Could you check a few things on this model? Use its own coordinates, in mm. A direction names the side the tool comes from. Coordinates: 2 decimals unless noted, no trailing zeros. Loops run counter-clockwise (first coordinate to the right, second up) from the corner with the lowest first, then second, coordinate; pieces in that order, holes last.
from build123d import *

# Parameters (mm, degrees)
SKETCH1_R           = 34
SKETCH1_R_2         = 31.5
BOSS_EXTRUDE1_DEPTH = 13
SKETCH2_R           = 34
BOSS_EXTRUDE2_DEPTH = 3
FILLET1_R           = 3
SKETCH3_R           = 2.5
SKETCH3_R_2         = 1.5
BOSS_EXTRUDE3_DEPTH = 10
SKETCH5_R           = 32.5
SKETCH5_R_2         = 31.5
CUT_EXTRUDE1_DEPTH  = 3
SKETCH6_R           = 1.6
CUT_EXTRUDE2_DEPTH  = 0.4
SKETCH7_R           = 1.5
CUT_EXTRUDE3_DEPTH  = 16.6


with BuildPart() as part:
    # Sketch1 → Boss-Extrude1 (new body)
    with BuildSketch(Plane.XY):
        Circle(SKETCH1_R)
        Circle(SKETCH1_R_2, mode=Mode.SUBTRACT)
    extrude(amount=BOSS_EXTRUDE1_DEPTH)

    # Sketch2 → Boss-Extrude2 (add)
    with BuildSketch(Plane.XY.offset(13)):
        Circle(SKETCH2_R)
    extrude(amount=BOSS_EXTRUDE2_DEPTH)

    # Fillet1
    fillet1_edges = [part.edges().sort_by_distance(p)[0] for p in [
        (-34, 0, 16),
    ]]
    fillet(fillet1_edges, radius=FILLET1_R)

    # Sketch3 → Boss-Extrude3 (add)
    with BuildSketch(Plane(origin=(0, 0, 13), x_dir=(-1, 0, 0), z_dir=(0, 0, -1))):
        with Locations((-20, 0)):
            Circle(SKETCH3_R)
        with Locations((-20, 0)):
            Circle(SKETCH3_R_2, mode=Mode.SUBTRACT)
        with Locations((20, 0)):
            Circle(SKETCH3_R)
        with Locations((20, 0)):
            Circle(SKETCH3_R_2, mode=Mode.SUBTRACT)
    extrude(amount=BOSS_EXTRUDE3_DEPTH)

    # Sketch5 → Cut-Extrude1 (cut)
    with BuildSketch(Plane(origin=(0, 0, 0), x_dir=(-1, 0, 0), z_dir=(0, 0, -1))):
        Circle(SKETCH5_R)
        Circle(SKETCH5_R_2, mode=Mode.SUBTRACT)
    extrude(amount=-CUT_EXTRUDE1_DEPTH, mode=Mode.SUBTRACT)

    # Sketch6 → Cut-Extrude2 (cut)
    with BuildSketch(Plane.XY.offset(16)):
        with Locations((0, -25)):
            Circle(SKETCH6_R)
    extrude(amount=-CUT_EXTRUDE2_DEPTH, mode=Mode.SUBTRACT)

    # Sketch7 → Cut-Extrude3 (cut, through all)
    with BuildSketch(Plane.XY.offset(15.6)):
        with Locations((0, -25)):
            Circle(SKETCH7_R)
    extrude(amount=-CUT_EXTRUDE3_DEPTH, mode=Mode.SUBTRACT)


solid = part.part
(1) For pin 1 (4 mm diameter, centred on x = -20, y = 0, fed in from -Z); pin 2 (19.5 mm diameter, centred on x = 3, y = 11, fed in from -Z); pin 3 (1.5 mm diameter, centred on x = 9.5, z = 3, fed in from -Y), each with a flat end and sliding along its axis, tell me the tip position at first contact or that it passes through.
Answers:
pin 1: stops at z = 3
pin 2: stops at z = 13
pin 3: stops at y = -32.85
(2) Imagine slicing it at C-C, the plane z = 1.75. Write out the boundary of the cut face in (x, y), and give its area (3 significant figures).
Answers:
outline: circle Ø68 at (0, 0); hole circle Ø65 at (0, 0)
area: 313 mm2
(3) Imagine slicing it at A-A, the plane z = 9.5. Write out the boundary of the cut face in (x, y), and give its area (3 significant figures).
Answers:
outline: circle Ø68 at (0, 0); circle Ø5 at (-20, 0); circle Ø5 at (20, 0); hole circle Ø63 at (0, 0); hole circle Ø3 at (-20, 0); hole circle Ø3 at (20, 0)
area: 540 mm2
(4) Which directions (+Z, -Z, +X, -X, +Y, -Y) give clear straight access to the entire face, cutting with the end or side of a thin tool? Please do faces 1 (the face through (0, 0, 13)), 2 (the face through (-0.195, -23.513, 14.318)), 3 (the face through (-0.208, -23.414, 15.803)).
Answers:
face 1: -Z
face 2: +Z, -Z
face 3: +Z
(5) We'd pull the mould along X, two halves only. Please class faces 4 (the face through (18.28, 28.67, 6.41)), 5 (the face through (0, 0, 16)), 6 (the face through (-17.5, 0.1, 8.1)): +X half, -X half, draft (parallel to the pull), parting line (faces both ways), or undercut.
Answers:
face 4: parting line
face 5: draft
face 6: undercut
(6) I need wall thicknesses on probe 1 along Y at (x, z) = (0, 1.05); probe 2 along Y at (x, z) = (-19, 9.75); probe 3 along Z at (x, y) = (4.5, -21.5). Which ranges of each line are inside material? Lowest first, please.
Answers:
probe 1: y = -34 to -32.5, 32.5 to 34
probe 2: y = -28.2 to -25.12, -2.29 to -1.12, 1.12 to 2.29, 25.12 to 28.2
probe 3: z = 13 to 16
(7) Imagine slicing it at D-D, the plane z = 14. Write out the boundary of the cut face in (x, y), and give its area (3 significant figures).
Answers:
outline: circle Ø67.66 at (0, 0); hole circle Ø3 at (0, -25)
area: 3,590 mm2
